from build123d import *

# Parameters (mm, degrees)
F0_R     = 7.874
F1_DEPTH = 10.922
F0_W     = 52.578
F0_H     = 10.922
F2_DEPTH = 44.45
F3_SIZE2 = 33.1422148526
F3_SIZE  = 16.5711074262
F4_SIZE2 = 52.567648
F4_SIZE  = 33.52799


# Not quite as in the source:
# - a fillet or chamfer is up to 0.001 mm smaller than in the source, because OpenCascade refuses the exact size


with BuildPart() as f1:
    # F0 (on Right) → F1 (new body)
    with BuildSketch(Plane.YZ):
        Polygon((-41.4015134737, 34.2036390094), (-73.1515134737, 34.2036390094), (-73.1515134737, 20.6804594447), (-62.2295134737, 20.6804594447), (-62.2295134737, -19.1975405553), (-9.6515134737, -19.1975405553), (-9.6515134737, -30.1195405553), (41.1484865263, -30.1195405553), (41.1484865263, 12.0844331742), align=None)
        with Locations((22.0984865263, -9.0175536905)):
            Circle(F0_R, mode=Mode.SUBTRACT)
    extrude(amount=F1_DEPTH)

    # F0 (on Right) → F2 (join)
    with BuildSketch(Plane.YZ):
        with Locations((-35.9405134737, -24.6585405553)):
            Rectangle(F0_W, F0_H)
        Polygon((-62.2295134737, 20.6804594447), (-73.1515134737, 20.6804594447), (-73.1515134737, -30.1195405553), (-62.2295134737, -30.1195405553), (-62.2295134737, -19.1975405553), align=None)
    extrude(amount=F2_DEPTH)

    # F3
    f3_edges = [f1.edges().sort_by_distance(p)[0] for p in [
        (44.45, -67.690513, 20.680459),
    ]]
    f3_side = f1.faces().sort_by_distance((27.686, -67.690513, 20.680459))[0]
    chamfer(f3_edges, length=F3_SIZE, length2=F3_SIZE2, reference=f3_side)

    # F4 (size 33.528 and 52.5676582111 in the source; OpenCascade refuses exactly that, so slightly less here)
    f4_edges = [f1.edges().sort_by_distance(p)[0] for p in [
        (44.45, -9.651513, -24.658541),
    ]]
    f4_side = f1.faces().sort_by_distance((27.686, -9.651513, -24.658541))[0]
    chamfer(f4_edges, length=F4_SIZE, length2=F4_SIZE2, reference=f4_side)


solid = f1.part
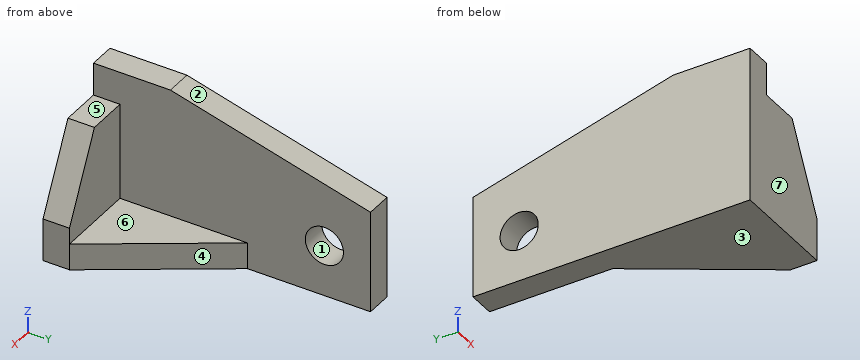
Can you work these out from the model? Positions are in its coordinate system, mm. Face numbers are marked on the shaded views. A direction names the side the tool comes from. Give positions to 0.01 mm unless a question says otherwise; leave off trailing zeros. Loops run counter-clockwise (first coordinate to the right, second up) from the corner with the lowest first, then second, coordinate; pieces in that order, holes last. Notation, with made-up numbers: (-2, 73) - (5, 73) arc R16 cw to (5, 90) - close; hole circle Ø6 at (55.25, 79.5). An arc over 180 degrees is marked (long way). Return JSON: item names as keys, results as strings.
1. I want a section at A-A on y = 18. Please give me the cut outline in (x, z).
Output values:
{"outline": "(0, -30.12) - (10.92, -30.12) - (10.92, -15.74) - (0, -15.74) - close; (0, -2.29) - (10.92, -2.29) - (10.92, 18.29) - (0, 18.29) - close"}
2. I'm going to push flat-ended pins straight in: pin 1 Ø1 at (y, z) = (-19.5, 26.5) entering from +X; pin 2 Ø10 at (x, z) = (28, 4) entering from +Y; pin 3 Ø3 at (x, y) = (10, -8.5) entering from +Z; pin 4 Ø10 at (y, z) = (-47, -21.5) entering from -X. Where does each tip first touch, or does it pass through?
Output values:
{"pin 1": "stops at x = 10.92", "pin 2": "stops at y = -62.23", "pin 3": "stops at z = 25.79", "pin 4": "stops at x = 0"}
3. I want a section at C-C on x = 5. Please give me the cut outline in (y, z), and give its area (3 significant figures).
Output values:
{"outline": "(-73.15, -30.12) - (41.15, -30.12) - (41.15, 12.08) - (-41.4, 34.2) - (-73.15, 34.2) - close; hole circle Ø15.75 at (22.1, -9.02)", "area": "6,240 mm²"}
4. For the marked faces 5, 6 and 7, which set-ups out of +Z, -Z, +X, -X, +Y, -Y let a thin tool reach every point of the face, with its end or its side?
Output values:
{"face 5": "+Z, +X, +Y, -Y", "face 6": "+Z, +X, +Y", "face 7": "+Z, -Z, +X, -X, -Y"}
5. We'd pull the mould along Z, two halves only. Please class the marked faces 1, 2, 3 and 4: +Z half, -Z half, draft (parallel to the pull), parting line (faces both ways), or undercut.
Output values:
{"face 1": "undercut", "face 2": "+Z half", "face 3": "-Z half", "face 4": "draft"}
6. If I drill on line 1 (Z direction, x = 16, y = -33); line 2 (X direction, y = -36, z = 3.5); line 3 (Y direction, x = 39.5, z = -15.5), over which ranges is the centre line in solid material (lowest first)?
Output values:
{"line 1": "z = -30.12 to -19.2", "line 2": "x = 0 to 10.92", "line 3": "y = -73.15 to -62.23"}
7. I want a section at B-B on z = -7. Please give me the cut outline in (x, y).
Output values:
{"outline": "(0, -73.15) - (41.72, -73.15) - (41.72, -62.23) - (10.92, -62.23) - (10.92, 14.49) - (0, 14.49) - close; (0, 29.71) - (10.92, 29.71) - (10.92, 41.15) - (0, 41.15) - close"}
